Input: dimensioned drawing with shaded views. Units: mm. Origin: part minimum x, y, z. A direction names the side the tool comes from. Coordinates: 2 decimals unless noted, no trailing zeros. Loops run counter-clockwise (first coordinate to the right, second up) from the corner with the lowest first, then second, coordinate; pieces in that order, holes last.
Item 1: Reachability of the marked faces 1, 2 and 3 from +Z, -Z, +X, -X, +Y, -Y: full face, straight path, thin tool, end or side. Return the list, or none.
Item 2: Section C-C on z = 185. Return loops of the section in (x, y).
Item 3: Section A-A on x = 10. Return loops of the section in (y, z).
Item 4: Section D-D on y = 33. Return loops of the section in (x, z).
Item 5: Contact query for flat-ended pins moving along their axis: P1, Ø4, axis at x = 11, z = 22, coming from the +Y side; P2, Ø11.5, axis at x = 10, y = 33, coming from the -Z side; P3, Ø12, axis at x = 13, y = 26.5, coming from the +Z side. Output: stop coordinate, or through.
Item 6: Section B-B on y = 10. Return loops of the section in (x, z), and give its area (3 significant figures).
Item 7: Ray query, line 1 along Z through (x, y) = (18.5, 26); line 2 along Z through (x, y) = (8.5, 9.5) (3 decimals); line 3 along Y through (x, z) = (2, 85.5). Return the intervals inside material, ascending.
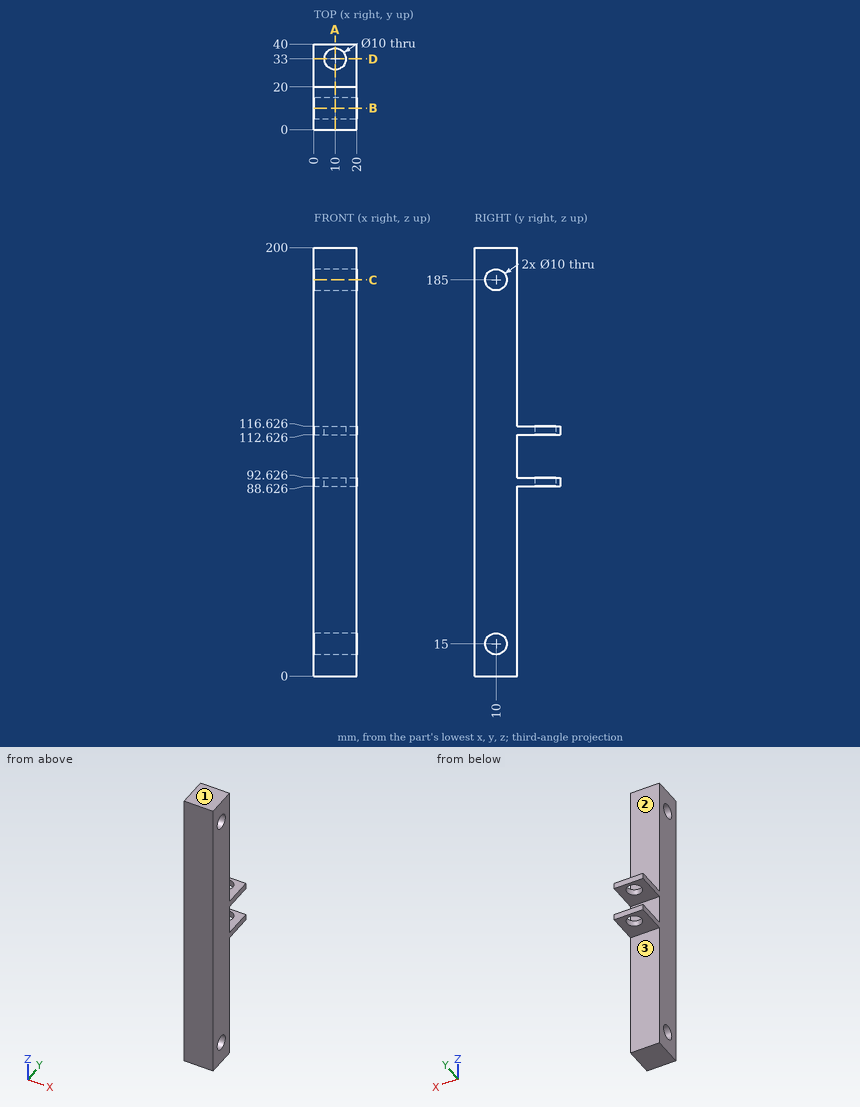
Results found:
1. face 1: +Z, +X, -X, +Y, -Y
1. face 2: +Z, +X, -X, +Y
1. face 3: -Z, +X, -X, +Y
2. outline: (0, 0) - (20, 0) - (20, 5) - (0, 5) - close; (0, 15) - (20, 15) - (20, 20) - (0, 20) - close
3. outline: (0, 0) - (20, 0) - (20, 88.63) - (28, 88.63) - (28, 92.63) - (20, 92.63) - (20, 112.63) - (28, 112.63) - (28, 116.63) - (20, 116.63) - (20, 200) - (0, 200) - close; (38, 88.63) - (40, 88.63) - (40, 92.63) - (38, 92.63) - close; (38, 112.63) - (40, 112.63) - (40, 116.63) - (38, 116.63) - close; hole circle Ø10 at (10, 15); hole circle Ø10 at (10, 185)
4. outline: (0, 88.63) - (5, 88.63) - (5, 92.63) - (0, 92.63) - close; (0, 112.63) - (5, 112.63) - (5, 116.63) - (0, 116.63) - close; (15, 88.63) - (20, 88.63) - (20, 92.63) - (15, 92.63) - close; (15, 112.63) - (20, 112.63) - (20, 116.63) - (15, 116.63) - close
5. P1: stops at y = 20
5. P2: stops at z = 88.63
5. P3: stops at z = 116.63
6. outline: (0, 0) - (20, 0) - (20, 10) - (0, 10) - close; (0, 20) - (20, 20) - (20, 180) - (0, 180) - close; (0, 190) - (20, 190) - (20, 200) - (0, 200) - close
6. area: 3,600 mm2
7. line 1: z = 88.63 to 92.63, 112.63 to 116.63
7. line 2: z = 0 to 10.025, 19.975 to 180.025, 189.975 to 200
7. line 3: y = 0 to 20
